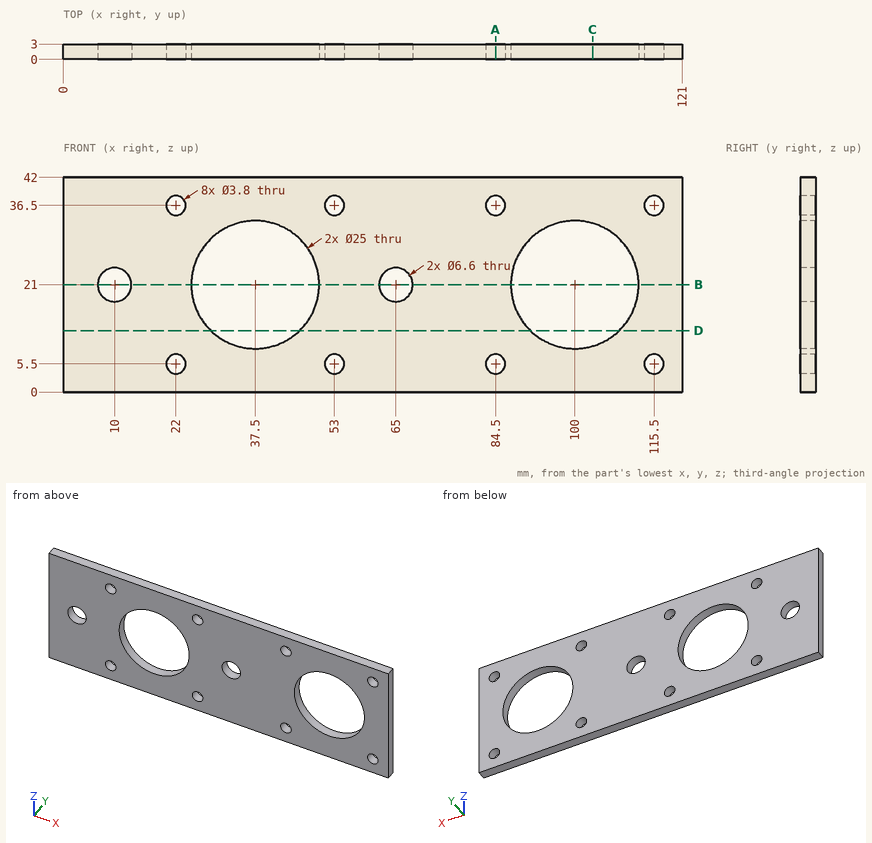
Drawing for the job (mm, zero at the part's lowest x, y, z). Round coordinates to 2 decimals unless told otherwise and drop trailing zeros. Write each loop counter-clockwise with the first axis right and the second up, starting at its lowest first coordinate (ties: lowest second). Pieces come first, ordered by that corner, then holes. Notation, with made-up numbers: (38, 83) - (77, 83) arc R29 cw to (77, 114) - close; hole circle Ø8 at (-3.75, 46). An arc over 180 degrees is marked (long way). Return JSON: item names as keys, results as strings. Group by question number.
Item 1: Band-saw the part on C-C on x = 103.5. List the corners of the cut face in (y, z).
Item 2: Band-saw the part on D-D on z = 12. List the corners of the cut face in (x, y).
Item 3: Band-saw the part on A-A on x = 84.5. List the corners of the cut face in (y, z), plus the area to 3 significant figures.
Item 4: Probe probe 1 along Z at (x, y) = (22, 1.25); probe 2 along X at (y, z) = (1.2, 36.5); probe 3 along X at (y, z) = (0.55, 20). List the from-to ranges inside material, lowest first.
Item 5: Flat gauge pin, fed straight in: pin 1 Ø2 at (x, z) = (51, 14.5) entering from -Y. Where does the tip first touch, or does it go through?
Item 6: Band-saw the part on B-B on z = 21. List the corners of the cut face in (x, y).
Resolved:
{
 "1": {"outline": "(0, 0) - (3, 0) - (3, 9) - (0, 9) - close; (0, 33) - (3, 33) - (3, 42) - (0, 42) - close"},
 "2": {"outline": "(0, 0) - (28.83, 0) - (28.83, 3) - (0, 3) - close; (46.17, 0) - (91.33, 0) - (91.33, 3) - (46.17, 3) - close; (108.67, 0) - (121, 0) - (121, 3) - (108.67, 3) - close"},
 "3": {"outline": "(0, 0) - (3, 0) - (3, 3.6) - (0, 3.6) - close; (0, 7.4) - (3, 7.4) - (3, 34.6) - (0, 34.6) - close; (0, 38.4) - (3, 38.4) - (3, 42) - (0, 42) - close", "area": "103 mm²"},
 "4": {"probe 1": "z = 0 to 3.6, 7.4 to 34.6, 38.4 to 42", "probe 2": "x = 0 to 20.1, 23.9 to 51.1, 54.9 to 82.6, 86.4 to 113.6, 117.4 to 121", "probe 3": "x = 0 to 6.86, 13.14 to 25.04, 49.96 to 61.86, 68.14 to 87.54, 112.46 to 121"},
 "5": {"pin 1": "stops at y = 0"},
 "6": {"outline": "(0, 0) - (6.7, 0) - (6.7, 3) - (0, 3) - close; (13.3, 0) - (25, 0) - (25, 3) - (13.3, 3) - close; (50, 0) - (61.7, 0) - (61.7, 3) - (50, 3) - close; (68.3, 0) - (87.5, 0) - (87.5, 3) - (68.3, 3) - close; (112.5, 0) - (121, 0) - (121, 3) - (112.5, 3) - close"}
}
